from build123d import *

# Parameters (mm, degrees)
F0_R     = 5.5372
F1_DEPTH = 50.8
F2_R     = 9.525
F3_DEPTH = 120.65
F4_SIZE  = 2.54
F5_SIZE  = 1.27


with BuildPart() as f1:
    # F0 (on Top) → F1 (new body)
    with BuildSketch(Plane.XY):
        Circle(F0_R)
    extrude(amount=F1_DEPTH)

    # F2 (on face) → F3 (join)
    with BuildSketch(Plane.XY.offset(50.8)):
        Circle(F2_R)
    extrude(amount=F3_DEPTH)

    # F4
    f4_edges = [f1.edges().sort_by_distance(p)[0] for p in [
        (-9.525, 0, 171.45),
    ]]
    chamfer(f4_edges, length=F4_SIZE)

    # F5
    f5_edges = [f1.edges().sort_by_distance(p)[0] for p in [
        (-9.525, 0, 50.8),
    ]]
    chamfer(f5_edges, length=F5_SIZE)


solid = f1.part
Here's how the part is built. I have some questions about the finished solid (model axes, mm). A direction names the side the tool comes from. Give positions to 0.01 mm unless a question says otherwise; leave off trailing zeros. Loops run counter-clockwise (first coordinate to the right, second up) from the corner with the lowest first, then second, coordinate; pieces in that order, holes last. Notation, with made-up numbers: (-7, 8) -> (32, 8) arc R14 ccw to (32, 17) -> close; hole circle Ø3 at (78.25, 1.5). An arc over 180 degrees is marked (long way). Answer as a JSON object with one key per item and string values. Group by question number.
Item 1: On a 3-axis mill with a long thin cutter (end or side, diameter ignored), from which of +Z, -Z, +X, -X, +Y, -Y can I reach the whole of each face in a straight line? I mean faces 1 (the cylindrical face through (-7.559, -5.796, 109.672)), 2 (the flat face through (-2, -5.4, 50.8)). Say none if no direction works.
Item 2: Will these pins go through, and if not, where does the flat tip stop? pin 1 (1 mm diameter, centred on y = 4.5, z = 114, fed in from +X); pin 2 (6 mm diameter, centred on x = 7, y = -5.5, fed in from -Z); pin 3 (1.5 mm diameter, centred on y = 3.5, z = 129.5, fed in from -X).
Item 3: Imagine slicing it at C-C on z = 159. Write out the boundary of the cut face in (x, y) (3 decimals).
Item 4: I need wall thicknesses on L1, parallel to X at y = 4.75, z = 76; L2, parallel to X at y = 7.75, z = 151.5; L3, parallel to Z at x = 6.5, y = 2. Which ranges of each line are inside material? Lowest first, please.
Item 5: Imagine slicing it at A-A on x = 0. Write out the boundary of the cut face in (y, z) (3 decimals), then the cut area to 3 significant figures.
Answer list:
{
 "1": {"face 1": "+Z, -Z", "face 2": "-Z"},
 "2": {"pin 1": "stops at x = 8.64", "pin 2": "stops at z = 50.8", "pin 3": "stops at x = -9.12"},
 "3": {"outline": "circle Ø19.05 at (0, 0)"},
 "4": {"L1": "x = -8.26 to 8.26", "L2": "x = -5.54 to 5.54", "L3": "z = 50.8 to 171.45"},
 "5": {"outline": "(-9.525, 52.07) -> (-8.255, 50.8) -> (-5.537, 50.8) -> (-5.537, 0) -> (5.537, 0) -> (5.537, 50.8) -> (8.255, 50.8) -> (9.525, 52.07) -> (9.525, 168.91) -> (6.985, 171.45) -> (-6.985, 171.45) -> (-9.525, 168.91) -> close", "area": "2,850 mm2"}
}
